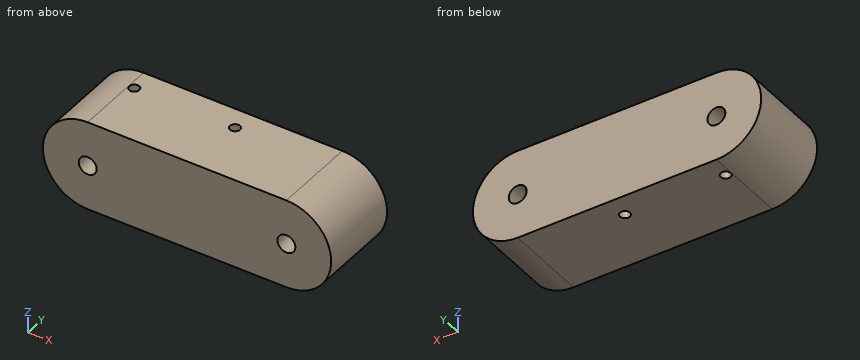
```python
from build123d import *

# Parameters (mm, degrees)
SKETCH_1_R          = 1.6
EXTRUDE_1_DEPTH     = 15
SKETCH_2_R          = 0.9
CUT_EXTRUDE_1_DEPTH = 49.716013794


with BuildPart() as part:
    # 草图1 → 凸台-拉伸1 (new body)
    with BuildSketch(Plane(origin=(0, 0, 0), x_dir=(1, 0, 0), z_dir=(0, 1, 0))):
        with BuildLine():
            Line((0, 8), (35.5, 8))
            ThreePointArc((35.5, 8), (43.5, 0), (35.5, -8))
            Line((35.5, -8), (0, -8))
            ThreePointArc((0, -8), (-8, 0), (0, 8))
        make_face()
        with Locations(Location((35.5, 0, 0), (0, 0, 270))):
            Circle(SKETCH_1_R, mode=Mode.SUBTRACT)
        with Locations(Location((0, 0, 0), (0, 0, 270))):
            Circle(SKETCH_1_R, mode=Mode.SUBTRACT)
    extrude(amount=EXTRUDE_1_DEPTH)

    # 草图2 → 切除-拉伸1 (cut, through all)
    with BuildSketch(Plane.XY.offset(8)):
        with Locations((19, 11)):
            Circle(SKETCH_2_R)
        with Locations((1, 11)):
            Circle(SKETCH_2_R)
    extrude(amount=-CUT_EXTRUDE_1_DEPTH, mode=Mode.SUBTRACT)


solid = part.part
```
Could you check a few things on this model? Use its own coordinates, in mm. Round coordinates to 2 decimals unless told otherwise and drop trailing zeros. Write each loop counter-clockwise with the first axis right and the second up, starting at its lowest first coordinate (ties: lowest second). Pieces come first, ordered by that corner, then holes. Notation, with made-up numbers: M -12,-22 L 47,-22 A19 cw 47,-5 Z; hole C 24.25,73.25 d1. An arc over 180 degrees is marked long. Answer in a Markdown table with one row per item. Add a question column.
Q1. Imagine slicing it at A-A (x = 19). Please give me the cut outline in (y, z).
Q2. Imagine slicing it at C-C (y = 11). Please give me the cut outline in (x, z), then the cut area to 3 significant figures.
Q3. Will these pins go through, and if not, where does the flat tip stop? pin 1 Ø2 at (y, z) = (3.5, 3) entering from -X; pin 2 Ø6 at (y, z) = (9, 4.5) entering from -X.
Q4. Imagine slicing it at D-D (x = 1). Please give me the cut outline in (y, z).
Q5. Imagine slicing it at B-B (z = 0). Please give me the cut outline in (x, y).
Q6. If I drill on line 1 (X direction, y = 6.75, z = 0); line 2 (X direction, y = 3, z = 1); line 3 (Y direction, x = 19, z = 4.75), over which ranges is the centre line in solid material (lowest first)? Write a range as from..to.
Values:
| question | item | result |
|---|---|---|
| 1 | outline | M 0,-8 L 10.1,-8 L 10.1,8 L 0,8 Z; M 11.9,-8 L 15,-8 L 15,8 L 11.9,8 Z |
| 2 | outline | M 0,-8 L 0.1,-8 L 0.1,-1.6 A1.6 cw long 0.1,1.6 L 0.1,8 L 0,8 A8 ccw Z; M 1.9,-8 L 18.1,-8 L 18.1,8 L 1.9,8 Z; M 19.9,-8 L 35.5,-8 A8 ccw 35.5,8 L 19.9,8 Z; hole C 35.5,0 d3.2 |
| 2 | area | 699 mm^2 |
| 3 | pin 1 | x = -7.75 |
| 3 | pin 2 | x = -7.86 |
| 4 | outline | M 0,-8 L 10.1,-8 L 10.1,-1.25 L 0,-1.25 Z; M 0,1.25 L 10.1,1.25 L 10.1,8 L 0,8 Z; M 11.9,-8 L 15,-8 L 15,-1.25 L 11.9,-1.25 Z; M 11.9,1.25 L 15,1.25 L 15,8 L 11.9,8 Z |
| 5 | outline | M -8,0 L -1.6,0 L -1.6,15 L -8,15 Z; M 1.6,0 L 33.9,0 L 33.9,15 L 1.6,15 L 1.6,11.67 A0.9 cw 1.6,10.33 Z; M 37.1,0 L 43.5,0 L 43.5,15 L 37.1,15 Z; hole C 19,11 d1.8 |
| 6 | line 1 | -8..-1.6, 1.6..33.9, 37.1..43.5 |
| 6 | line 2 | -7.94..-1.25, 1.25..34.25, 36.75..43.44 |
| 6 | line 3 | 0..10.1, 11.9..15 |
